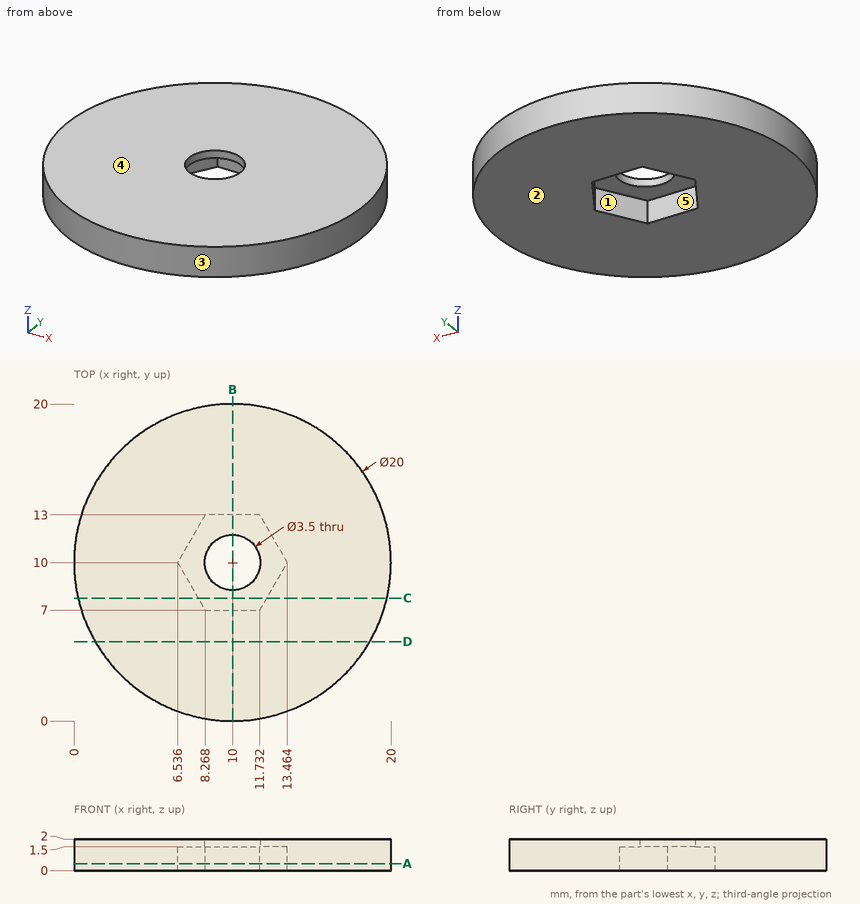
Could you check a few things on this drawing? It's one solid part, dimensions in mm from its lowest x, y, z. A direction names the side the tool comes from. Give positions to 0.01 mm unless a question says otherwise; leave off trailing zeros. Write each loop counter-clockwise with the first axis right and the second up, starting at its lowest first coordinate (ties: lowest second). Pieces come first, ordered by that corner, then holes.
(1) Imagine slicing it at C-C, the plane y = 7.75. Write out the boundary of the cut face in (x, z) (1 decimal), and give its area (3 significant figures).
Output values:
outline: (0.3, 0) - (7.8, 0) - (7.8, 1.5) - (12.2, 1.5) - (12.2, 0) - (19.7, 0) - (19.7, 2) - (0.3, 2) - close
area: 32.5 mm2
(2) Imagine slicing it at D-D, the plane y = 5. Write out the boundary of the cut face in (x, z).
Output values:
outline: (1.34, 0) - (18.66, 0) - (18.66, 2) - (1.34, 2) - close
(3) On a 3-axis mill with a long thin cutter (end or side, diameter ignored), from which of +Z, -Z, +X, -X, +Y, -Y can I reach the whole of each face in a straight line? I mean the marked faces 1 and 2. Say none if no direction works.
Output values:
face 1: -Z
face 2: -Z, +X, -X, +Y, -Y
(4) Will these pins go through, and if not, where does the flat tip stop? pin 1 (1.8 mm diameter, centred on x = 11, y = 9.5, fed in from -Z); pin 2 (1.2 mm diameter, centred on x = 11, z = 1, fed in from +Y).
Output values:
pin 1: stops at z = 1.5
pin 2: stops at y = 19.99
(5) If I drill on L1, parallel to Y at x = 10, z = 1.7; L2, parallel to X at y = 10.5, z = 0.9 (1 decimal); L3, parallel to Z at x = 11.5, y = 9, over which ranges is the centre line in solid material (lowest first)?
Output values:
L1: y = 0 to 8.25, 11.75 to 20
L2: x = 0 to 6.8, 13.2 to 20
L3: z = 1.5 to 2
(6) Imagine slicing it at B-B, the plane x = 10. Write out the boundary of the cut face in (y, z).
Output values:
outline: (0, 0) - (7, 0) - (7, 1.5) - (8.25, 1.5) - (8.25, 2) - (0, 2) - close; (11.75, 1.5) - (13, 1.5) - (13, 0) - (20, 0) - (20, 2) - (11.75, 2) - close
(7) Imagine slicing it at A-A, the plane z = 0.45. Write out the boundary of the cut face in (x, y).
Output values:
outline: circle Ø20 at (10, 10); hole (6.54, 10) - (8.27, 7) - (11.73, 7) - (13.46, 10) - (11.73, 13) - (8.27, 13) - close
(8) Thinking about a two-plate mould opening in X: for the marked faces 3, 4 and 5, which applies, pulls with the +X half, pulls with the -X half, needs draft (parallel to the pull), parting line crosses it, or undercut?
Output values:
face 3: parting line crosses it
face 4: needs draft
face 5: undercut
